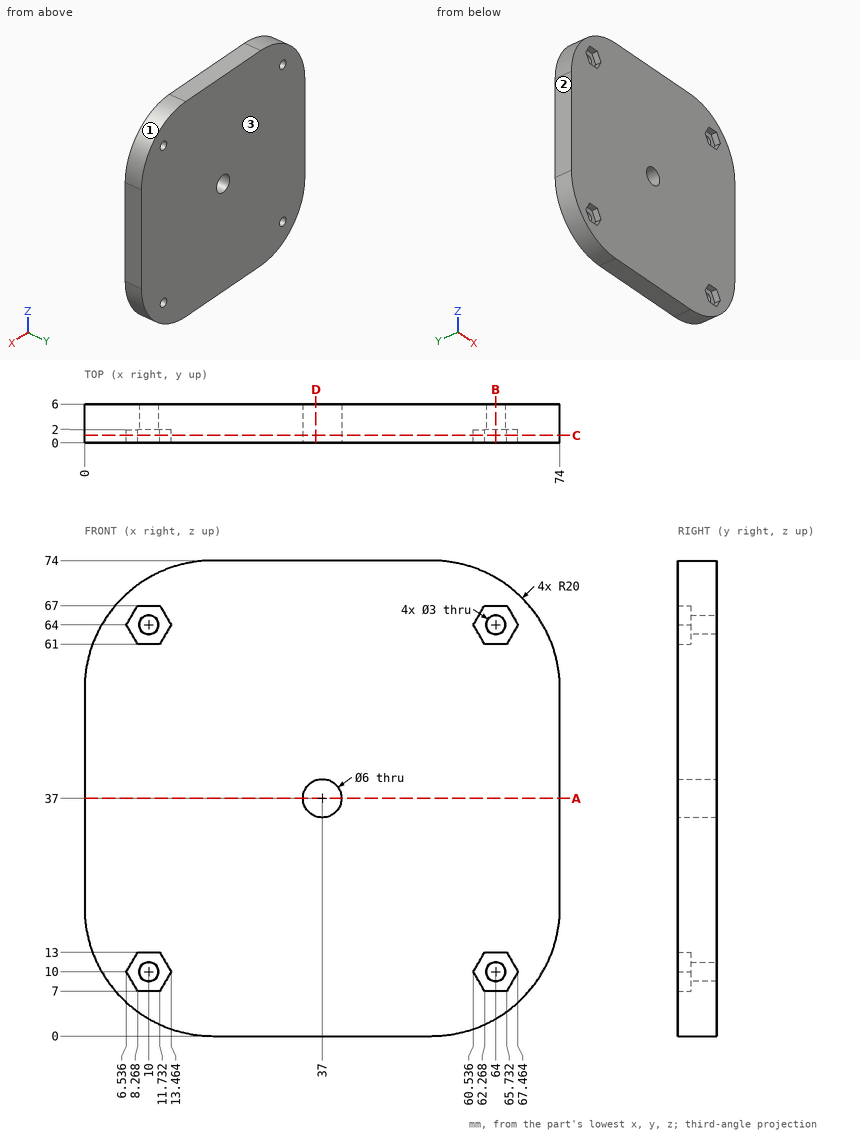
Input: dimensioned drawing with shaded views. Units: mm. Origin: part minimum x, y, z. Give positions to 0.01 mm unless a question says otherwise; leave off trailing zeros. Loops run counter-clockwise (first coordinate to the right, second up) from the corner with the lowest first, then second, coordinate; pieces in that order, holes last. Notation, with made-up numbers: (-1, -3) - (38, -3) arc R25 cw to (38, 32) - close; hole circle Ø7 at (34.5, -25). An arc over 180 degrees is marked (long way). Answer as CSV lines item,"result". Start each with the question number.
(1) Section query B-B (x = 64). Output: boundary loops of the cut face in (y, z).
(2) Pin query (flat end, axial travel): P1, Ø0.6, axis at x = 64, y = 1, coming from the +Z side; P2, Ø5.5, axis at x = 37, z = 37, coming from the +Y side; P3, Ø2, axis at x = 64.5, y = 1, coming from the +Z side; P4, Ø5, axis at x = 11, z = 11, coming from the -Y side. Return the tip coordinate at first contact, or that it passes through.
(3) Mould query, pull axis X, two halves, no side actions, for the marked faces 1, 2 and 3. Classes: +X half, -X half, draft (parallel to the pull), parting line (faces both ways), or undercut.
(4) Ray query, line 1 along X through (y, z) = (3.8, 10); line 2 along X through (y, z) = (2.5, 37). Return the intervals inside material, ascending. Write a range as [from, to].
(5) Section query A-A (z = 37). Output: boundary loops of the cut face in (x, y), and give its area (3 significant figures).
(6) Section query C-C (y = 1.1). Give the number of separate pieces and of enclosed holes in the cut face, and give its area (3 significant figures).
(7) Section query D-D (x = 36). Output: boundary loops of the cut face in (y, z), and give its area (3 significant figures).
Worked answers:
1,outline,"(0, 2.68) - (6, 2.68) - (6, 8.5) - (2, 8.5) - (2, 7) - (0, 7) - close; (0, 13) - (2, 13) - (2, 11.5) - (6, 11.5) - (6, 62.5) - (2, 62.5) - (2, 61) - (0, 61) - close; (0, 67) - (2, 67) - (2, 65.5) - (6, 65.5) - (6, 71.32) - (0, 71.32) - close"
2,P1,"stops at z = 71.49"
2,P2,"passes through"
2,P3,"stops at z = 71.6"
2,P4,"stops at y = 0"
3,face 1,"+X half"
3,face 2,"-X half"
3,face 3,"draft"
4,line 1,"x = [2.68, 8.5], [11.5, 62.5], [65.5, 71.32]"
4,line 2,"x = [0, 34], [40, 74]"
5,outline,"(0, 0) - (34, 0) - (34, 6) - (0, 6) - close; (40, 0) - (74, 0) - (74, 6) - (40, 6) - close"
5,area,"408 mm^2"
6,separate pieces,"1"
6,enclosed holes,"5"
6,area,"4,980 mm^2"
7,outline,"(0, 0) - (6, 0) - (6, 34.17) - (0, 34.17) - close; (0, 39.83) - (6, 39.83) - (6, 74) - (0, 74) - close"
7,area,"410 mm^2"
